Here's how the part is built. I have some questions about the finished solid (model axes, mm). A direction names the side the tool comes from. Round coordinates to 2 decimals unless told otherwise and drop trailing zeros. Loops run counter-clockwise (first coordinate to the right, second up) from the corner with the lowest first, then second, coordinate; pieces in that order, holes last. Notation, with made-up numbers: M -22.75,12 L 19.25,12 A18 cw 19.25,47 Z; hole C 5,0.25 d7. An arc over 180 degrees is marked long. Use a Markdown table: item, result.
Autodesk Fusion 360 part; units mm, degrees
sketch "Sketch1" plane through (0, 0, 0) normal (0, 1, 0) x (1, 0, 0)
  circle A0 centre (0, 0) radius 25
  circle A1 centre (-13, 0) radius 3
  circle A2 centre (13, 0) radius 3
  circle A3 centre (-13, 0) radius 5.5
  circle A4 centre (13, 0) radius 5.5
  circle A5 centre (0, 0) radius 18.25
  dimension "d1" = 50
  dimension "d2" = 26
  dimension "d3" = 13
  dimension "d4" = 6
  dimension "d5" = 6
  dimension "d17" = 11
  dimension "d18" = 11
  dimension "d41" = 36.5
extrude "Extrude1" add sketch "Sketch1" along normal blind 8 contours A0 | A3 A5 | A3 A4 A5 | A3 A5 | A4 A5 | A4 A5
sketch "Sketch2" plane through (0, 8, 0) normal (0, 1, 0) x (-1, 0, 0)
  circle A0 centre (13, 0) radius 3
  circle A1 centre (-13, 0) radius 3
  circle A2 centre (0, 0) radius 3
  circle A3 centre (0, 0) radius 25
  circle A4 centre (0, 0) radius 6.3
  dimension "d26" = 6
  dimension "d37" = 12.6
hole "Hole1" at (0, 8, 0) direction (0, -1, 0) diameter 6.2 depth 9 tip angle 118 counterbore diameter 12.4 counterbore depth 6
extrude "Extrude2" cut sketch "Sketch1" along normal blind 5.5 contours A3 A5 | A3 A5 | A4 A5 | A4 A5
extrude "Extrude4" cut sketch "Sketch1" along normal blind 2.7 contours A0
chamfer "Chamfer1" distance 1 angle 45 1 edges at (-23.3082, 8, 9.0404)
fillet "Fillet1" radius 2 4 edges at (-18.1466, 1.35, 1.9396) (-18.1466, 1.35, -1.9396) (18.1466, 1.35, 1.9396) (18.1466, 1.35, -1.9396)
sketch "Sketch3" plane through (0, 0, 0) normal (0, -1, 0) x (1, 0, 0)
  arc A0 (16.2765, -8.2545) -> (14.0947, -5.39) centre (14.4928, -7.3499) ccw
  arc A1 (14.0947, 5.39) -> (14.0947, -5.39) centre (13, 0) ccw
  arc A2 (14.0947, 5.39) -> (16.2765, 8.2545) centre (14.4928, 7.3499) ccw
  arc A3 (16.2765, 8.2545) -> (-16.2765, 8.2545) centre (0, 0) ccw
  arc A4 (-16.2765, 8.2545) -> (-14.0947, 5.39) centre (-14.4928, 7.3499) ccw
  arc A5 (-14.0947, -5.39) -> (-14.0947, 5.39) centre (-13, 0) ccw
  arc A6 (-14.0947, -5.39) -> (-16.2765, -8.2545) centre (-14.4928, -7.3499) ccw
  arc A7 (-16.2765, -8.2545) -> (16.2765, -8.2545) centre (0, 0) ccw
  circle A8 centre (0, 0) radius 3.1
  circle A9 centre (0, 0) radius 18.25
  dimension "d46" = 36.5
sketch "Sketch4" plane through (0, 0, 0) normal (0, -1, 0) x (1, 0, 0)
  arc A0 (16.2765, -8.2545) -> (14.0947, -5.39) centre (14.4928, -7.3499) ccw
  arc A1 (14.0947, 5.39) -> (14.0947, -5.39) centre (13, 0) ccw
  arc A2 (14.0947, 5.39) -> (16.2765, 8.2545) centre (14.4928, 7.3499) ccw
  arc A3 (16.2765, 8.2545) -> (-16.2765, 8.2545) centre (0, 0) ccw
  arc A4 (-16.2765, 8.2545) -> (-14.0947, 5.39) centre (-14.4928, 7.3499) ccw
  arc A5 (-14.0947, -5.39) -> (-14.0947, 5.39) centre (-13, 0) ccw
  arc A6 (-14.0947, -5.39) -> (-16.2765, -8.2545) centre (-14.4928, -7.3499) ccw
  arc A7 (-16.2765, -8.2545) -> (16.2765, -8.2545) centre (0, 0) ccw
  circle A8 centre (0, 0) radius 3.1
  line L0 (30, 27.5) -> (-30, 27.5)
  line L1 (-30, 27.5) -> (-30, -27.5)
  line L2 (-30, -27.5) -> (30, -27.5)
  line L3 (30, -27.5) -> (30, 27.5)
  line L4 (30, 27.5) -> (-30, -27.5) construction
  line L5 (-30, 27.5) -> (30, -27.5) construction
  dimension "d47" = 60
  dimension "d48" = 55
equation "d3 = d2 / 2"
Q1. I need wall thicknesses on line 1 (Z direction, x = 0, y = 0.9); line 2 (X direction, y = 2.05, z = 0); line 3 (Y direction, x = 18.5, z = 5). Which ranges of each line are inside material? Lowest first, please. Write a range as from..to.
Return value:
| item | result |
|---|---|
| line 1 | z = -18.25..-3.1, 3.1..18.25 |
| line 2 | x = -7.5..-6.2, 6.2..7.5 |
| line 3 | y = 2.7..8 |
Q2. We'd pull the mould along X, two halves only. Please class faces 1 (the cylindrical face through (0.281, 1.331, 18.248)), 2 (the cylindrical face through (-16, 7, 0)), 3 (the flat face through (16, 2.7, 5)): pulls with the +X half, pulls with the -X half, needs draft (parallel to the pull), parting line crosses it, or undercut.
Return value:
| item | result |
|---|---|
| face 1 | parting line crosses it |
| face 2 | undercut |
| face 3 | needs draft |
Q3. Imagine slicing it at B-B, the plane z = 0. Give the number of separate pieces and of enclosed holes in the cut face, then the cut area to 3 significant figures.
Return value:
| item | result |
|---|---|
| separate pieces | 4 |
| enclosed holes | 0 |
| area | 126 mm^2 |
Q4. Imagine slicing it at A-A, the plane x = 0. Please give me the cut outline in (y, z), then the cut area to 3 significant figures.
Return value:
| item | result |
|---|---|
| outline | M 0,-18.25 L 2.7,-18.25 L 2.7,-25 L 7,-25 L 8,-24 L 8,-6.2 L 2,-6.2 L 2,-3.1 L 0,-3.1 Z; M 0,3.1 L 2,3.1 L 2,6.2 L 8,6.2 L 8,24 L 7,25 L 2.7,25 L 2.7,18.25 L 0,18.25 Z |
| area | 276 mm^2 |
Q5. Imagine slicing it at C-C, the plane y = 4. Please give me the cut outline in (x, z), then the cut area to 3 significant figures.
Return value:
| item | result |
|---|---|
| outline | C 0,0 d50; hole C -13,0 d11; hole C 0,0 d12.4; hole C 13,0 d11 |
| area | 1,650 mm^2 |
Q6. For faces 4 (the flat face through (5, 8, 5)), 5 (the cylindrical face through (-7.754, 3.323, 1.652)), 6 (the cylindrical face through (5.5, 4.96, 2.86)), 7 (the cylindrical face through (-0.281, 1.331, -18.248)), 8 (the cylindrical face through (23.846, 4.82, 7.509)), which set-ups out of +Z, -Z, +X, -X, +Y, -Y let a thin tool reach every point of the face, with its end or its side?
Return value:
| item | result |
|---|---|
| face 4 | +Z, -Z, +X, -X, +Y |
| face 5 | -Y |
| face 6 | +Y |
| face 7 | -Z, -Y |
| face 8 | +Y, -Y |
Q7. Will these pins go through, and if not, where does the flat tip stop? P1, Ø3.5, axis at x = 2.5, z = -3, coming from the +Y side; P2, Ø1.5, axis at y = 3.5, z = -3, coming from the +X side; P3, Ø10, axis at x = -18, z = 16.5, coming from the -Y side; P4, Ø3.5, axis at x = -13, z = 0, coming from the +Y side.
Return value:
| item | result |
|---|---|
| P1 | stops at y = 2 |
| P2 | stops at x = 24.9 |
| P3 | stops at y = 2.7 |
| P4 | passes through |
